The figure shows three views and two pictorial views of one solid part (mm, origin at its lowest corner). Answer the questions. Round coordinates to 2 decimals unless told otherwise and drop trailing zeros. Order: outer loops, then holes, each group sorted by start corner. A loop starts at its lowest first (then second) coordinate and runs counter-clockwise, first axis right, second up. Notation, with made-up numbers: M 39,63 L 85,63 A17 ccw 85,92 Z; hole C -24,66 d5. An arc over 180 degrees is marked long. Return JSON: item names as keys, results as strings.
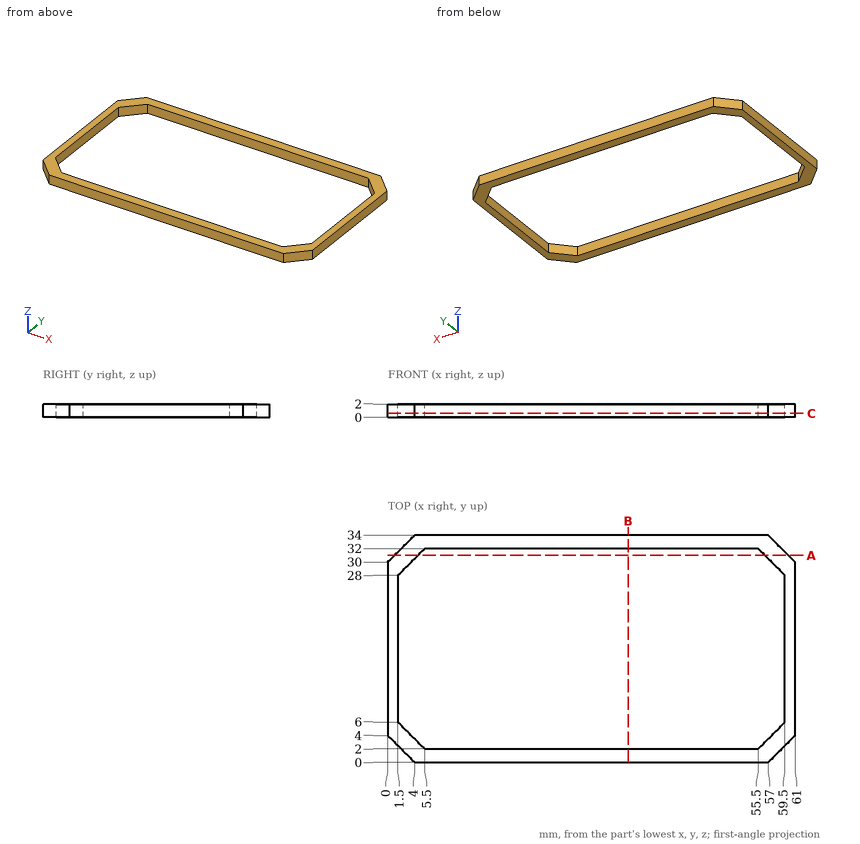
Item 1: Find section B-B (x = 36). Determine the outline of the cut face in (y, z), plus the area to 3 significant figures.
Output:
{"outline": "M 0,0 L 2,0 L 2,2 L 0,2 Z; M 32,0 L 34,0 L 34,2 L 32,2 Z", "area": "8.00 mm^2"}
Item 2: Find section A-A (y = 31). Determine the outline of the cut face in (x, z), plus the area to 3 significant figures.
Output:
{"outline": "M 1,0 L 4.5,0 L 4.5,2 L 1,2 Z; M 56.5,0 L 60,0 L 60,2 L 56.5,2 Z", "area": "14.0 mm^2"}
Item 3: Find section C-C (z = 0.6). Determine the outline of the cut face in (x, y), plus the area to 3 significant figures.
Output:
{"outline": "M 0,4 L 4,0 L 57,0 L 61,4 L 61,30 L 57,34 L 4,34 L 0,30 Z; hole M 1.5,6 L 5.5,2 L 55.5,2 L 59.5,6 L 59.5,28 L 55.5,32 L 5.5,32 L 1.5,28 Z", "area": "334 mm^2"}
Item 4: Consider line 1 along X through (y, z) = (12.5, 1.05); line 2 along Y through (x, z) = (11.5, 1.1); line 3 along Y through (x, z) = (4, 1.85). Determine where each line is inside the solid, lowest interval first. Write a range as [from, to].
Output:
{"line 1": "x = [0, 1.5], [59.5, 61]", "line 2": "y = [0, 2], [32, 34]", "line 3": "y = [0, 3.5], [30.5, 34]"}
